```python
from build123d import *

# Parameters (mm, degrees)
SKETCH1_W           = 115
SKETCH1_H           = 60
SKETCH1_R           = 2.1
BOSS_EXTRUDE1_DEPTH = 5
SKETCH2_R           = 4.575
CUT_EXTRUDE1_DEPTH  = 3
SKETCH3_R           = 3.25
CUT_EXTRUDE2_DEPTH  = 0.2
SKETCH4_R           = 1.65
CUT_EXTRUDE3_DEPTH  = 6
CUT_EXTRUDE4_DEPTH  = 6
BOSS_EXTRUDE2_DEPTH = 5
SKETCH8_R           = 1.65
CUT_EXTRUDE5_DEPTH  = 6
FILLET1_R           = 5
SKETCH9_R           = 6
SKETCH9_R_2         = 2.1
BOSS_EXTRUDE3_DEPTH = 2.275
SKETCH10_R          = 2.9
SKETCH10_R_2        = 2.1
BOSS_EXTRUDE4_DEPTH = 0.2
SKETCH11_R          = 3
CUT_EXTRUDE6_DEPTH  = 1


with BuildPart() as part:
    # Sketch1 → Boss-Extrude1 (new body)
    with BuildSketch(Plane(origin=(0, 0, 0), x_dir=(1, 0, 0), z_dir=(0, 1, 0))):
        with Locations((-12.5, 0)):
            Rectangle(SKETCH1_W, SKETCH1_H)
        with Locations((-22, 14)):
            Circle(SKETCH1_R, mode=Mode.SUBTRACT)
        with Locations((0, 18)):
            Circle(SKETCH1_R, mode=Mode.SUBTRACT)
        with Locations((0, -18)):
            Circle(SKETCH1_R, mode=Mode.SUBTRACT)
        with Locations((-22, -14)):
            Circle(SKETCH1_R, mode=Mode.SUBTRACT)
        with Locations((15, -18)):
            Circle(SKETCH1_R, mode=Mode.SUBTRACT)
    extrude(amount=BOSS_EXTRUDE1_DEPTH)

    # Sketch2 → Cut-Extrude1 (cut)
    with BuildSketch(Plane(origin=(0, 5, 0), x_dir=(1, 0, 0), z_dir=(0, 1, 0))):
        Circle(SKETCH2_R)
    extrude(amount=-CUT_EXTRUDE1_DEPTH, mode=Mode.SUBTRACT)

    # Sketch3 → Cut-Extrude2 (cut)
    with BuildSketch(Plane(origin=(0, 2, 0), x_dir=(1, 0, 0), z_dir=(0, 1, 0))):
        Circle(SKETCH3_R)
    extrude(amount=-CUT_EXTRUDE2_DEPTH, mode=Mode.SUBTRACT)

    # Sketch4 → Cut-Extrude3 (cut, through all)
    with BuildSketch(Plane(origin=(0, 5, 0), x_dir=(1, 0, 0), z_dir=(0, 1, 0))):
        with Locations((-34.5, -8)):
            Circle(SKETCH4_R)
        with Locations((-34.5, 8)):
            Circle(SKETCH4_R)
    extrude(amount=-CUT_EXTRUDE3_DEPTH, mode=Mode.SUBTRACT)

    # Sketch6 → Cut-Extrude4 (cut, through all)
    with BuildSketch(Plane(origin=(0, 5, 0), x_dir=(1, 0, 0), z_dir=(0, 1, 0))):
        with BuildLine():
            Line((-22, 18.221576202), (-34.5, 18.221576202))
            ThreePointArc((-34.5, 18.221576202), (-38.035533906, 16.757110108), (-39.5, 13.221576202))
            Line((-39.5, 13.221576202), (-39.5, -13.221576202))
            ThreePointArc((-39.5, -13.221576202), (-38.035533906, -16.757110108), (-34.5, -18.221576202))
            Line((-34.5, -18.221576202), (-22, -18.221576202))
            Line((-22, -18.221576202), (-8.297519941, -18.221576202))
            Line((-8.297519941, -18.221576202), (0.548980681, -18.221576202))
            Line((0.548980681, -18.221576202), (26.801199277, -38.580439602))
            Line((26.801199277, -38.580439602), (-22, -30))
            Line((-22, -30), (-70, -30))
            Line((-70, -30), (-70, 30))
            Line((-70, 30), (-22, 30))
            Line((-22, 30), (26.801199277, 38.580439602))
            Line((26.801199277, 38.580439602), (0.548980681, 18.221576202))
            Line((0.548980681, 18.221576202), (-8.297519941, 18.221576202))
            Line((-8.297519941, 18.221576202), (-22, 18.221576202))
        make_face()
    extrude(amount=-CUT_EXTRUDE4_DEPTH, mode=Mode.SUBTRACT)

    # Sketch7 → Boss-Extrude2 (add)
    with BuildSketch(Plane(origin=(0, 5, 0), x_dir=(1, 0, 0), z_dir=(0, 1, 0))):
        Polygon((27.342211368, 39), (15.73694821, 30), (45, 30), (45, 39), align=None)
        Polygon((45, -30), (15.73694821, -30), (27.342211368, -39), (45, -39), align=None)
    extrude(amount=-BOSS_EXTRUDE2_DEPTH)

    # Sketch8 → Cut-Extrude5 (cut, through all)
    with BuildSketch(Plane(origin=(0, 5, 0), x_dir=(1, 0, 0), z_dir=(0, 1, 0))):
        with Locations((35, 32)):
            Circle(SKETCH8_R)
        with Locations((35, -32)):
            Circle(SKETCH8_R)
    extrude(amount=-CUT_EXTRUDE5_DEPTH, mode=Mode.SUBTRACT)

    # Fillet1
    fillet1_edges = [part.edges().sort_by_distance(p)[0] for p in [
        (45, 2.5, -39),
        (27.342211368, 2.5, -39),
        (27.342211368, 2.5, 39),
        (45, 2.5, 39),
    ]]
    fillet(fillet1_edges, radius=FILLET1_R)

    # Sketch9 → Boss-Extrude3 (add)
    with BuildSketch(Plane(origin=(0, 5, 0), x_dir=(1, 0, 0), z_dir=(0, 1, 0))):
        with Locations((15, -18)):
            Circle(SKETCH9_R)
        with Locations((15, -18)):
            Circle(SKETCH9_R_2, mode=Mode.SUBTRACT)
    extrude(amount=BOSS_EXTRUDE3_DEPTH)

    # Sketch10 → Boss-Extrude4 (add)
    with BuildSketch(Plane(origin=(0, 7.275, 0), x_dir=(1, 0, 0), z_dir=(0, 1, 0))):
        with Locations((15, -18)):
            Circle(SKETCH10_R)
        with Locations((15, -18)):
            Circle(SKETCH10_R_2, mode=Mode.SUBTRACT)
    extrude(amount=BOSS_EXTRUDE4_DEPTH)

    # Sketch11 → Cut-Extrude6 (cut)
    with BuildSketch(Plane(origin=(0, 5, 0), x_dir=(1, 0, 0), z_dir=(0, 1, 0))):
        with Locations((-34.5, 8)):
            Circle(SKETCH11_R)
        with Locations((-34.5, -8)):
            Circle(SKETCH11_R)
        with Locations((35, -32)):
            Circle(SKETCH11_R)
        with Locations((35, 32)):
            Circle(SKETCH11_R)
    extrude(amount=-CUT_EXTRUDE6_DEPTH, mode=Mode.SUBTRACT)


solid = part.part
```
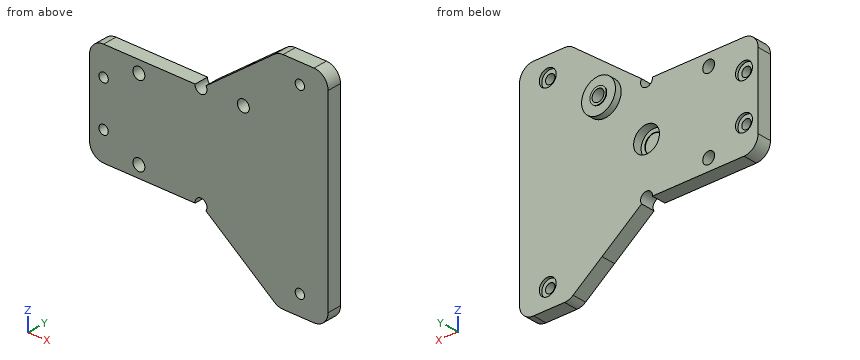
Input: part model. Units: mm. Frame: model coordinates. Coordinates: 2 decimals unless noted, no trailing zeros. Write each loop counter-clockwise with the first axis right and the second up, starting at its lowest first coordinate (ties: lowest second). Pieces come first, ordered by that corner, then holes.
1) Section C-C on z = 32. Output: boundary loops of the cut face in (x, y), and give its area (3 significant figures).
2) Section A-A on y = 6.25. Output: boundary loops of the cut face in (x, z), and give its area (3 significant figures).
3) Material intervals for line 1 along Z through (x, y) = (35, 4.3); line 2 along Z through (x, y) = (35, 2.8); line 3 along Z through (x, y) = (0, 1.9), sorted ascending.
4) Section D-D on x = 22. Output: boundary loops of the cut face in (y, z), and give its area (3 significant figures).
5) Pin query (flat end, axial travel): pin 1 Ø2.5 at (x, z) = (15, 18) entering from +Y; pin 2 Ø3 at (x, z) = (-35.5, 8.5) entering from +Y; pin 3 Ø5 at (x, z) = (0, -18) entering from +Y; pin 4 Ø2 at (y, z) = (3, -26) entering from -X. Return the tip coordinate at first contact, or that it passes through.
6) Section B-B on x = 0. Output: boundary loops of the cut face in (y, z) (3 decimals), and give its area (3 significant figures).
Check result:
1. outline: (18.32, 0) - (33.35, 0) - (33.35, 4) - (32, 4) - (32, 5) - (18.32, 5) - close; (36.65, 0) - (45, 0) - (45, 5) - (38, 5) - (38, 4) - (36.65, 4) - close
1. area: 114 mm2
2. outline: circle Ø12 at (15, 18); hole circle Ø4.2 at (15, 18)
2. area: 99.2 mm2
3. line 1: z = -39 to -35, -29 to 29, 35 to 39
3. line 2: z = -39 to -33.65, -30.35 to 30.35, 33.65 to 39
3. line 3: z = -15.9 to -3.25, 3.25 to 15.9
4. outline: (0, -34.86) - (5, -34.86) - (5, 34.86) - (0, 34.86) - close
4. area: 349 mm2
5. pin 1: passes through
5. pin 2: stops at y = 4
5. pin 3: stops at y = 5
5. pin 4: stops at x = 9.29
6. outline: (0, -15.9) - (5, -15.9) - (5, -4.575) - (2, -4.575) - (2, -3.25) - (1.8, -3.25) - (1.8, 3.25) - (2, 3.25) - (2, 4.575) - (5, 4.575) - (5, 15.9) - (0, 15.9) - close
6. area: 130 mm2
